from build123d import *

# Parameters (mm, degrees)
SKETCH1_W                       = 73.025
SKETCH1_H                       = 28.575
BOSS_EXTRUDE1_DEPTH             = 5.2740052
SKETCH2_W                       = 14.2875
SKETCH2_H                       = 0.762
CUT_EXTRUDE1_DEPTH              = 47.663780517
F_9_32_0_28125_DIAMETER_HOLE1_D = 7.14375
CHAMFER1_SIZE                   = 0.635
CHAMFER2_SIZE                   = 0.635


with BuildPart() as part:
    # Sketch1 → Boss-Extrude1 (new body)
    with BuildSketch(Plane(origin=(0, 0, 0), x_dir=(1, 0, 0), z_dir=(0, 1, 0))):
        Rectangle(SKETCH1_W, SKETCH1_H)
    extrude(amount=BOSS_EXTRUDE1_DEPTH)

    # Sketch2 → Cut-Extrude1 (cut, through all)
    with BuildSketch(Plane.XY.offset(14.2875)):
        with Locations((-29.36875, 0.381)):
            Rectangle(SKETCH2_W, SKETCH2_H)
        with Locations((29.36875, 0.381)):
            Rectangle(SKETCH2_W, SKETCH2_H)
    extrude(amount=-CUT_EXTRUDE1_DEPTH, mode=Mode.SUBTRACT)

    # 9/32 (0.28125) Diameter Hole1 (through all)
    with Locations(Plane(origin=(0, 5.2740052, 0), x_dir=(-1, 0, 0), z_dir=(0, 1, 0))):
        with Locations((27, -7.5), (-27, 7.5), (-27, -7.5), (27, 7.5)):
            Hole(F_9_32_0_28125_DIAMETER_HOLE1_D / 2)

    # Chamfer1
    chamfer1_edges = [part.edges().sort_by_distance(p)[0] for p in [
        (36.5125, 3.0180026, 14.2875),
        (-36.5125, 3.0180026, 14.2875),
        (-36.5125, 3.0180026, -14.2875),
        (36.5125, 3.0180026, -14.2875),
    ]]
    chamfer(chamfer1_edges, length=CHAMFER1_SIZE)

    # Chamfer2
    chamfer2_edges = [part.edges().sort_by_distance(p)[0] for p in [
        (-30.571875, 5.2740052, 7.5),
        (23.428125, 5.2740052, -7.5),
        (23.428125, 5.2740052, 7.5),
        (-30.571875, 5.2740052, -7.5),
        (36.5125, 5.2740052, 0),
        (0, 5.2740052, 14.2875),
        (0, 5.2740052, -14.2875),
        (-36.5125, 5.2740052, 0),
        (-36.195, 5.2740052, 13.97),
        (-36.195, 5.2740052, -13.97),
        (36.195, 5.2740052, -13.97),
        (36.195, 5.2740052, 13.97),
    ]]
    chamfer(chamfer2_edges, length=CHAMFER2_SIZE)


solid = part.part
For this review, take the finished solid that the model builds, in its own axes (mm). A direction names the side the tool comes from. Give positions to 0.01 mm unless a question says otherwise; leave off trailing zeros. Order: outer loops, then holes, each group sorted by start corner. A loop starts at its lowest first (then second) coordinate and runs counter-clockwise, first axis right, second up. Notation, with made-up numbers: M 73,61 L 83,61 A12 ccw 83,73 Z; hole C 61,80.25 d2. An arc over 180 degrees is marked long. Answer in a Markdown table with one row per item. Add a question column.
(1) Consider section D-D on z = 1.25. State the section outline as (x, y) points (1 decimal).
(2) Consider section A-A on x = 27. State the section outline as (y, z) points.
(3) Consider section B-B on z = 7.5. State the section outline as (x, y) points (1 decimal), and give its area (3 significant figures).
(4) Mouldability with a two-part tool opening along X and no side actions: class faces 3 (the face through (-23.7, 2.67, 6.13)), 4 (the face through (-23.7, 2.67, -8.87)), 5 (the face through (-29, 0.762, 0)), 6 (the face through (36.512, 3, 0)) as +X half, -X half, draft (parallel to the pull), parting line (faces both ways), or undercut.
(5) Consider section C-C on y = 2.15. State the section outline as (x, z) points.
(6) Wall thickness on probe 1 along Z at (x, y) = (-27, 3.5); probe 2 along Z at (x, y) = (24.5, 1.7); probe 3 along X at (y, z) = (2.3, 9.5): over which ranges is each line inside the solid? List them lowest first. Write a range as [from, to].
(7) For faces 1 (the face through (-1, 2, -14.288)), 2 (the face through (29, 0.762, 0)), list the 3-axis set-ups (+Z, -Z, +X, -X, +Y, -Y) from which the entire face can be reached by the end or side of a thin tool; tool diameter is ignored.
(8) For pin 1 (5.5 mm diameter, centred on x = -27, z = -7.5, fed in from -Y); pin 2 (1 mm diameter, centred on x = 10, z = -1.5, fed in from -Y); pin 3 (11.5 mm diameter, centred on x = -32, z = 1, fed in from -Y); pin 4 (0.6 mm diameter, centred on y = 0, z = -6, fed in from +X) (3 decimals), all flat-tipped, find the tip position at first contact; note any pin that passes through.
Evaluation:
| question | item | result |
|---|---|---|
| 1 | outline | M -36.5,0.8 L -22.2,0.8 L -22.2,0 L 22.2,0 L 22.2,0.8 L 36.5,0.8 L 36.5,4.6 L 35.9,5.3 L -35.9,5.3 L -36.5,4.6 Z |
| 2 | outline | M 0.76,-14.29 L 4.64,-14.29 L 5.27,-13.65 L 5.27,-11.71 L 4.64,-11.07 L 0.76,-11.07 Z; M 0.76,-3.93 L 4.64,-3.93 L 5.27,-3.29 L 5.27,3.29 L 4.64,3.93 L 0.76,3.93 Z; M 0.76,11.07 L 4.64,11.07 L 5.27,11.71 L 5.27,13.65 L 4.64,14.29 L 0.76,14.29 Z |
| 3 | outline | M -36.5,0.8 L -30.6,0.8 L -30.6,4.6 L -31.2,5.3 L -35.9,5.3 L -36.5,4.6 Z; M -23.4,0.8 L -22.2,0.8 L -22.2,0 L 22.2,0 L 22.2,0.8 L 23.4,0.8 L 23.4,4.6 L 22.8,5.3 L -22.8,5.3 L -23.4,4.6 Z; M 30.6,0.8 L 36.5,0.8 L 36.5,4.6 L 35.9,5.3 L 31.2,5.3 L 30.6,4.6 Z |
| 3 | area | 298 mm^2 |
| 4 | face 3 | undercut |
| 4 | face 4 | undercut |
| 4 | face 5 | draft |
| 4 | face 6 | +X half |
| 5 | outline | M -36.51,-13.65 L -35.88,-14.29 L 35.88,-14.29 L 36.51,-13.65 L 36.51,13.65 L 35.88,14.29 L -35.88,14.29 L -36.51,13.65 Z; hole C -27,-7.5 d7.14; hole C -27,7.5 d7.14; hole C 27,-7.5 d7.14; hole C 27,7.5 d7.14 |
| 6 | probe 1 | z = [-14.29, -11.07], [-3.93, 3.93], [11.07, 14.29] |
| 6 | probe 2 | z = [-14.29, -10.05], [-4.95, 4.95], [10.05, 14.29] |
| 6 | probe 3 | x = [-36.51, -29.96], [-24.04, 24.04], [29.96, 36.51] |
| 7 | face 1 | -Z, +X, -X, +Y, -Y |
| 7 | face 2 | +Z, -Z, +X, -Y |
| 8 | pin 1 | passes through |
| 8 | pin 2 | stops at y = 0 |
| 8 | pin 3 | stops at y = 0.76 |
| 8 | pin 4 | stops at x = 22.225 |
